Autodesk Inventor part; units mm, degrees
ref_plane "YZ Plane" through (0, 0, 0) normal (1, 0, 0) x (0, 1, 0)
ref_plane "XZ Plane" through (0, 0, 0) normal (0, 1, 0) x (-1, 0, 0)
ref_plane "XY Plane" through (0, 0, 0) normal (0, 0, 1) x (1, 0, 0)
sketch "Skizze2" plane through (0, 0, 0) normal (0, 1, 0) x (-1, 0, 0)
  line L0 (0, 0) -> (47.2, 0)
  line L1 (47.2, 0) -> (47.2, 21.85)
  line L2 (47.2, 21.85) -> (0, 21.85)
  line L3 (0, 21.85) -> (0, 0)
  dimension "d5" = 47.2
  dimension "d6" = 21.85
extrude "Extrusion2" add sketch "Skizze2" along normal blind 2.5
sketch "Skizze3" plane through (0, 0, 21.85) normal (1, 0, 0) x (0, 0, -1)
  line L0 (10.425, 3.5) -> (11.425, 3.5)
  line L1 (11.425, 3.5) -> (11.425, 2.5)
  line L2 (11.425, 2.5) -> (10.425, 2.5)
  line L3 (10.425, 2.5) -> (10.425, 3.5)
  line L4 (0, 2.5) -> (21.85, 2.5)
  point P0 (21.85, 0)
  point P1 (10.925, 2.5)
  point P2 (10.925, 2.5)
  point P3 (10.925, 2.5)
  dimension "d9" = 1
  dimension "d10" = 1
extrude "Extrusion3" add sketch "Skizze3" along normal blind 1 and the other way blind 11
sketch "Skizze4" plane through (-47.2, 0, 0) normal (-1, 0, 0) x (0, 0, 1)
  line L0 (4.925, 4.6) -> (16.925, 4.6)
  line L1 (16.925, 4.6) -> (16.925, 0)
  line L2 (16.925, 0) -> (4.925, 0)
  line L3 (4.925, 0) -> (4.925, 4.6)
  line L4 (0, 0) -> (21.85, 0)
  point P0 (10.925, 0)
  point P1 (10.925, 0)
  point P2 (10.925, 0)
  dimension "d15" = 12
  dimension "d16" = 4.6
extrude "Extrusion4" [suppressed]
sketch "Skizze5" plane through (0, 0, 0) normal (0, -1, 0) x (1, 0, 0)
  line L0 (-47.2, 17.425) -> (-41, 17.425)
  line L1 (-41, 17.425) -> (-41, 4.425)
  line L2 (-41, 4.425) -> (-47.2, 4.425)
  line L3 (-47.2, 4.425) -> (-47.2, 17.425)
  line L4 (-47.2, 16.925) -> (-61.7, 16.925)
  line L5 (-47.2, 4.925) -> (-61.7, 4.925)
  line L6 (0, 21.85) -> (0, 0)
  line L7 (-11.5, 19.85) -> (0, 19.85)
  line L8 (0, 19.85) -> (0, 2)
  line L9 (0, 2) -> (-11.5, 2)
  line L10 (-11.5, 2) -> (-11.5, 19.85)
  line L11 (-47.2, 21.85) -> (0, 21.85)
  line L12 (0, 0) -> (-47.2, 0)
  point P0 (0, 19.85)
  dimension "d21" = 6.2
  dimension "d22" = 13
  dimension "d23" = 0.5
  dimension "d24" = 0.5
  dimension "d25" = 11.5
  dimension "d26" = 2
  dimension "d27" = 2
extrude "Extrusion5" add sketch "Skizze5" along normal blind 1 contours L6 L9 L10 L7
ref_plane "Arbeitsebene1" through (-47.2, 0, 10.925) normal (0, 0, 1) x (1, 0, 0)
equation "\"d23\" = d24"
properties part number "hdmi grabber"
Input: part model. Units: mm. Frame: model coordinates. A direction names the side the tool comes from. Give positions to 0.01 mm unless a question says otherwise; leave off trailing zeros. Loops run counter-clockwise (first coordinate to the right, second up) from the corner with the lowest first, then second, coordinate; pieces in that order, holes last. Notation, with made-up numbers: (-22, -32.5) - (29, -32.5) arc R19 cw to (29, -19.5) - close; hole circle Ø7 at (60.25, -20.5). An arc over 180 degrees is marked (long way). Use CSV: the item, a comma, the result in double quotes. Start each with the question number.
Item 1: Section B-B on z = 17.25. Return loops of the section in (x, y), then the cut area to 4 significant figures.
Item 2: Section D-D on y = -0.45. Return loops of the section in (x, z), then the cut area to 3 significant figures.
Item 3: Section A-A on x = -8. Return loops of the section in (y, z) (3 decimals), then the cut area to 3 significant figures.
Item 4: Contact query for flat-ended pins moving along their axis: P1, Ø11, axis at x = -26, z = 10, coming from the -Y side; P2, Ø0.5, axis at x = 0.5, z = 11, coming from the -Y side; P3, Ø6.5, axis at x = -27.5, z = 13.5, coming from the +Y side. Output: stop coordinate, or through.
Item 5: Reachability of faces 1 (the flat face through (-5.7, -0.5, 2)), 2 (the flat face through (-5.8, -0.5, 19.85)), 3 (the flat face through (-5, 3, 11.425)), 4 (the flat face through (-11, 3, 11)) from +Z, -Z, +X, -X, +Y, -Y: full face, straight path, thin tool, end or side. Return the list, or none.
Item 6: Section C-C on y = 1.7. Return loops of the section in (x, z), then the cut area to 3 significant figures.
Item 7: Line query: line 1 (Y direction, x = -2, z = 11.5); line 2 (Y direction, x = -27.5, z = 12.75); line 3 (X direction, y = 0.8, z = 19). Output: solid intervals per line, ascending.
Ans:
1,outline,"(-47.2, 0) - (-11.5, 0) - (-11.5, -1) - (0, -1) - (0, 2.5) - (-47.2, 2.5) - close"
1,area,"129.5 mm2"
2,outline,"(-11.5, 2) - (0, 2) - (0, 19.85) - (-11.5, 19.85) - close"
2,area,"205 mm2"
3,outline,"(-1, 2) - (0, 2) - (0, 0) - (2.5, 0) - (2.5, 10.425) - (3.5, 10.425) - (3.5, 11.425) - (2.5, 11.425) - (2.5, 21.85) - (0, 21.85) - (0, 19.85) - (-1, 19.85) - close"
3,area,"73.5 mm2"
4,P1,"stops at y = 0"
4,P2,"stops at y = 2.5"
4,P3,"stops at y = 2.5"
5,face 1,"-Z, +X, -X, -Y"
5,face 2,"+Z, +X, -X, -Y"
5,face 3,"+Z, +X, -X, +Y"
5,face 4,"+Z, -Z, -X, +Y"
6,outline,"(-47.2, 0) - (0, 0) - (0, 21.85) - (-47.2, 21.85) - close"
6,area,"1,030 mm2"
7,line 1,"y = -1 to 2.5"
7,line 2,"y = 0 to 2.5"
7,line 3,"x = -47.2 to 0"
